Autodesk Fusion 360 part; units mm, degrees
sketch "Sketch1" plane through (0, 0, 0) normal (0, 0, 1) x (1, 0, 0)
  line L0 (0, 46.4728) -> (44.7124, 46.4728)
  line L1 (44.7124, 46.4728) -> (44.7124, 0.7041)
  line L2 (44.7124, 0.7041) -> (0, 0.7041)
  line L3 (0, 0.7041) -> (0, 46.4728)
  line L4 (34.7124, 10.7041) -> (10, 10.7041)
  line L5 (10, 10.7041) -> (10, 36.4728)
  line L6 (10, 36.4728) -> (34.7124, 36.4728)
  line L7 (34.7124, 36.4728) -> (34.7124, 10.7041)
  line L8 (22.3562, 46.4728) -> (22.3562, 0.7041) construction
  line L9 (0, 23.5884) -> (44.7124, 23.5884) construction
  line L10 (0, 22.0884) -> (44.7124, 22.0884)
  line L11 (0, 22.0884) -> (44.7124, 22.0884)
  line L12 (20.8562, 46.4728) -> (20.8562, 0.7041)
  line L13 (0, 25.0884) -> (44.7124, 25.0884)
  line L14 (23.8562, 46.4728) -> (23.8562, 0.7041)
  dimension "d1" = 10
  dimension "d2" = 1.5
  dimension "d3" = 1.5
extrude "Extrude1" add sketch "Sketch1" along normal blind 1.6 contours L0 L3 L5 L6 L12 L13 | L0 L1 L6 L7 L13 L14 | L5 L6 L12 L13 | L6 L12 L13 L14 | L2 L3 L4 L5 L10 L11 L12 | L5 L10 L11 L12 L13 | L6 L7 L13 L14 | L10 L11 L12 L13 L14 | L4 L5 L10 L11 L12 | L7 L10 L11 L13 L14 | L4 L10 L11 L12 L14 | L1 L2 L4 L7 L10 L11 L14 | L4 L7 L10 L11 L14
fillet "Fillet1" radius 3 5 edges at (0, 22.0884, 0.8) (0, 25.0884, 0.8) (20.8562, 0.7041, 0.8) (23.8562, 0.7041, 0.8) (44.7124, 25.0884, 0.8)
fillet "Fillet2" radius 3 3 edges at (23.8562, 46.4728, 0.8) (20.8562, 46.4728, 0.8) (44.7124, 22.0884, 0.8)
Read the model definition and answer for the solid it produces. Units are mm, in the model's axes. A direction names the side the tool comes from. Coordinates: 2 decimals unless noted, no trailing zeros. Order: outer loops, then holes, each group sorted by start corner. A loop starts at its lowest first (then second) coordinate and runs counter-clockwise, first axis right, second up. Notation, with made-up numbers: (-14, 74.5) - (29, 74.5) arc R21 ccw to (29, 112.5) - close; hole circle Ø6 at (38.5, -6.75). An arc over 180 degrees is marked (long way). Answer as a JSON object with one key per item and string values. Group by question number.
Item 1: Flat-ended cylindrical pins translate along their axes: P1, Ø0.8, axis at y = 24, z = 1, coming from the -X side; P2, Ø0.8, axis at x = 22.5, z = 1, coming from the +Y side. Find the tip coordinate at first contact, or state that the pin passes through.
Item 2: Section D-D (x = 22) is taken. Give the vertices of the cut face in (y, z), plus the area to 3 significant figures.
Item 3: Section B-B (y = 8) is taken. Give the vertices of the cut face in (x, z).
Item 4: Section C-C (z = 0.45) is taken. Give the vertices of the cut face in (x, y).
Item 5: Section A-A (x = 8) is taken. Give the vertices of the cut face in (y, z), plus the area to 3 significant figures.
Item 6: Consider probe 1 along X at (y, z) = (6, 0.65); probe 2 along Y at (x, z) = (5, 1.55); probe 3 along X at (y, z) = (44, 1). Determine where each line is inside the solid, lowest interval first. Write a range as from..to.
Item 7: The mould has two halves that part along Y. Classify faces 1 (the face through (10, 24, 1)), 2 (the face through (23.856, 40, 1)), 3 (the face through (36, 0.704, 1)): +Y half, -Y half, draft (parallel to the pull), parting line (faces both ways), or undercut.
Item 8: A tool of negligible diameter and unlimited length cuts with its end or side. For faces 4 (the face through (38, 22.088, 1)), 5 (the face through (6, 25.088, 1)), 6 (the face through (24.71, 1.61, 0.81)), from which of +Z, -Z, +X, -X, +Y, -Y can it reach the whole face along a straight path? Write none if from no direction.
Results are:
{
 "1": {"P1": "stops at x = 10", "P2": "stops at y = 36.47"},
 "2": {"outline": "(10.7, 0) - (36.47, 0) - (36.47, 1.6) - (10.7, 1.6) - close", "area": "41.2 mm^2"},
 "3": {"outline": "(0, 0) - (20.86, 0) - (20.86, 1.6) - (0, 1.6) - close; (23.86, 0) - (44.71, 0) - (44.71, 1.6) - (23.86, 1.6) - close"},
 "4": {"outline": "(0, 0.7) - (17.86, 0.7) arc R3 ccw to (20.86, 3.7) - (20.86, 10.7) - (23.86, 10.7) - (23.86, 3.7) arc R3 ccw to (26.86, 0.7) - (44.71, 0.7) - (44.71, 19.09) arc R3 ccw to (41.71, 22.09) - (34.71, 22.09) - (34.71, 25.09) - (41.71, 25.09) arc R3 ccw to (44.71, 28.09) - (44.71, 46.47) - (26.86, 46.47) arc R3 ccw to (23.86, 43.47) - (23.86, 36.47) - (20.86, 36.47) - (20.86, 43.47) arc R3 ccw to (17.86, 46.47) - (0, 46.47) - (0, 28.09) arc R3 ccw to (3, 25.09) - (10, 25.09) - (10, 22.09) - (3, 22.09) arc R3 ccw to (0, 19.09) - close"},
 "5": {"outline": "(0.7, 0) - (22.09, 0) - (22.09, 1.6) - (0.7, 1.6) - close; (25.09, 0) - (46.47, 0) - (46.47, 1.6) - (25.09, 1.6) - close", "area": "68.4 mm^2"},
 "6": {"probe 1": "x = 0..20.86, 23.86..44.71", "probe 2": "y = 0.7..22.09, 25.09..46.47", "probe 3": "x = 0..20.81, 23.9..44.71"},
 "7": {"face 1": "undercut", "face 2": "draft", "face 3": "-Y half"},
 "8": {"face 4": "+Z, -Z, +X", "face 5": "+Z, -Z, -X", "face 6": "+Z, -Z, -Y"}
}
